Autodesk Inventor part; units mm, degrees
ref_plane "YZ Plane" through (0, 0, 0) normal (1, 0, 0) x (0, 1, 0)
ref_plane "XZ Plane" through (0, 0, 0) normal (0, 1, 0) x (-1, 0, 0)
ref_plane "XY Plane" through (0, 0, 0) normal (0, 0, 1) x (1, 0, 0)
sketch "スケッチ1" plane through (0, 0, 0) normal (0, 0, 1) x (1, 0, 0)
  arc A0 (-5.1, 0) -> (5.1, 0) centre (0, 0) ccw
  line L0 (-15, 8) -> (15, 8)
  line L1 (15, 8) -> (15, 0)
  line L2 (15, 0) -> (5.1, 0)
  line L3 (-15, 0) -> (-15, 8)
  arc A1 (5.1, 0) -> (-5.1, 0) centre (0, 0) ccw
  line L4 (5.1, 0) -> (-5.1, 0)
  line L5 (-5.1, 0) -> (-15, 0)
  dimension "d0" = 10.2
  dimension "d1" = 30
  dimension "d2" = 15
  dimension "d3" = 8
  dimension "d4" = 0
extrude "押し出し1" add sketch "スケッチ1" along normal blind 30 contours L5 L3 L0 L1 L2 A1
sketch "スケッチ2" plane through (-15, 0, 0) normal (0, -1, 0) x (1, 0, 0)
  line L0 (9.9, 30) -> (0, 30)
  line L1 (0, 0) -> (9.9, 0)
  line L2 (0, 30) -> (4.95, 30)
  line L3 (4.95, 30) -> (4.95, 0)
  line L4 (4.95, 0) -> (0, 0)
  line L5 (0, 0) -> (0, 30)
  line L6 (30, 30) -> (25.05, 30)
  line L7 (25.05, 30) -> (25.05, 0)
  line L8 (25.05, 0) -> (30, 0)
  line L9 (30, 0) -> (30, 30)
  line L10 (4.95, 30) -> (9.9, 30)
  line L11 (9.9, 30) -> (9.9, 0)
  line L12 (9.9, 0) -> (4.95, 0)
  line L13 (4.95, 0) -> (4.95, 30)
  line L14 (25.05, 30) -> (20.1, 30)
  line L15 (20.1, 30) -> (20.1, 0)
  line L16 (20.1, 0) -> (25.05, 0)
  line L17 (25.05, 0) -> (25.05, 30)
  point P0 (15, 0)
  dimension "d7" = 30
  dimension "d8" = 4.95
  dimension "d34" = 4.95
extrude "押し出し2" add sketch "スケッチ2" along normal blind 2 contours L11 L1 L3 L0 | L7 L16 L15 L14
fillet "フィレット2" radius 1 4 edges at (-10.05, 0, 15) (-10.05, -2, 15) (10.05, 0, 15) (10.05, -2, 15)
sketch "スケッチ3" plane through (-15, 8, 0) normal (0, 1, 0) x (1, 0, 0)
  line L0 (0, -30) -> (30, -30)
  line L1 (30, 0) -> (30, -30)
  line L2 (30, 0) -> (0, 0)
  line L3 (0, 0) -> (0, -30)
  point P0 (15, 0)
  point P1 (5, -5)
  point P2 (5, -25)
  point P3 (25, -25)
  point P4 (25, -5)
  dimension "d11" = 5
  dimension "d12" = 5
  dimension "d13" = 5
  dimension "d14" = 5
  dimension "d15" = 5
  dimension "d16" = 5
  dimension "d17" = 5
  dimension "d18" = 5
hole "Hole3" at (-10, 8, 5) at (-10, 8, 25) at (10, 8, 25) at (10, 8, 5) direction (0, -1, 0) diameter 3 end through all
sketch "スケッチ4" plane through (0, 0, 30) normal (0, 0, 1) x (1, 0, 0)
  arc A0 (9.05, -2) -> (10.05, -1) centre (9.05, -1) ccw
  arc A1 (11.05, 0) -> (10.05, -1) centre (11.05, -1) ccw
  line L0 (15, 0) -> (11.05, 0)
  line L1 (15, 8) -> (15, 0)
  line L2 (-15, 8) -> (15, 8)
  line L3 (-15, 0) -> (-15, 8)
  line L4 (-11.05, 0) -> (-15, 0)
  arc A2 (-10.05, -1) -> (-11.05, 0) centre (-11.05, -1) ccw
  arc A3 (-10.05, -1) -> (-9.05, -2) centre (-9.05, -1) ccw
  line L5 (-9.05, -2) -> (-5.1, -2)
  line L6 (-5.1, 0) -> (-5.1, -2)
  arc A4 (5.1, 0) -> (-5.1, 0) centre (0, 0) ccw
  line L7 (5.1, 0) -> (5.1, -2)
  line L8 (5.1, -2) -> (9.05, -2)
  line L9 (-15, 0.1) -> (-10.95, 0.1)
  line L10 (-9.95, -0.9) -> (-9.95, -0.9)
  line L11 (-8.95, -1.9) -> (-5.1, -1.9)
  arc A5 (-9.95, -0.9) -> (-10.95, 0.1) centre (-10.95, -0.9) ccw
  arc A6 (-9.95, -0.9) -> (-8.95, -1.9) centre (-8.95, -0.9) ccw
  line L12 (0, 0) -> (0, 8)
  line L13 (15, 0.1) -> (10.95, 0.1)
  line L14 (8.95, -1.9) -> (5.1, -1.9)
  arc A7 (10.95, 0.1) -> (9.95, -0.9) centre (10.95, -0.9) ccw
  arc A8 (8.95, -1.9) -> (9.95, -0.9) centre (8.95, -0.9) ccw
  point P0 (-9.95, 0.1)
  dimension "d43" = 5.05
  dimension "d44" = 2.1
  dimension "d45" = 0.1
  dimension "d46" = 1
equation "\"d34\" = d8"
properties part number "poleHolderB" material "Aluminum-6061"
The listing builds one solid part. Answer for the finished solid, in the listing's coordinates (mm). A direction names the side the tool comes from. Round coordinates to 2 decimals unless told otherwise and drop trailing zeros. Order: outer loops, then holes, each group sorted by start corner. A loop starts at its lowest first (then second) coordinate and runs counter-clockwise, first axis right, second up. Notation, with made-up numbers: (-27.5, 38.5) - (6.5, 38.5) arc R27 cw to (6.5, 57.5) - close; hole circle Ø9 at (71, 16.5). An arc over 180 degrees is marked (long way). Put each result on its own line as item: value. Start each with the question number.
(1) Find section A-A (z = 5). Give the vertices of the cut face in (x, y).
(2) Straight lines are drawn through the part: probe 1 along X at (y, z) = (5.5, 5); probe 2 along Z at (x, y) = (-10, 5.5); probe 3 along X at (y, z) = (-1, 15.5). For each, find the intervals that lie inside material, in ascending order. Write a range as from..to.
(3) Find section B-B (y = 1). Give the vertices of the cut face in (x, z), plus the area to 3 significant figures.
(4) Given P1, Ø2.5, axis at x = 10, z = 25, coming from the -Y side; P2, Ø1.6, axis at y = -1, z = 9, coming from the -X side; P3, Ø4, axis at x = 1, z = 9.5, coming from the -Y side; P4, Ø1.2, axis at x = -14, z = 20.5, coming from the -Y side, each flat-ended and moving along its own axis, determine where each tip first touches the part or whether it passes through.
(5) Determine the mould class of faces 1 (the flat face through (-7, -2, 15)), 2 (the cylindrical face through (-0.1, 5.1, 14.8)), 3 (the cylindrical face through (9.765, -1.699, 14.876)) for opening direction X: released by +X, released by -X, zero draft, split by the parting line, or undercut.
(6) Find section C-C (y = 5.5). Give the vertices of the cut face in (x, z), plus the area to 3 significant figures.
(7) For faces 4 (the cylindrical face through (8.513, 2.93, 4.805)), 5 (the flat face through (-13, 0, 15)), determine the directions among +Z, -Z, +X, -X, +Y, -Y from which every point of the face is accessible in a straight line to the end or side of a thin tool.
Reply:
1. outline: (-15, 0) - (-11.5, 0) - (-11.5, 8) - (-15, 8) - close; (-8.5, -2) - (-5.1, -2) - (-5.1, 0) arc R5.1 cw to (5.1, 0) - (5.1, -2) - (8.5, -2) - (8.5, 8) - (-8.5, 8) - close; (11.5, 0) - (15, 0) - (15, 8) - (11.5, 8) - close
2. probe 1: -15..-11.5, -8.5..8.5, 11.5..15
2. probe 2: 0..3.5, 6.5..23.5, 26.5..30
2. probe 3: -10.05..-5.1, 5.1..10.05
3. outline: (-15, 0) - (-5, 0) - (-5, 30) - (-15, 30) - close; (5, 0) - (15, 0) - (15, 30) - (5, 30) - close; hole circle Ø3 at (-10, 5); hole circle Ø3 at (-10, 25); hole circle Ø3 at (10, 5); hole circle Ø3 at (10, 25)
3. area: 572 mm^2
4. P1: through
4. P2: x = -10.45
4. P3: y = 4.12
4. P4: y = 0
5. face 1: zero draft
5. face 2: undercut
5. face 3: released by +X
6. outline: (-15, 0) - (15, 0) - (15, 30) - (-15, 30) - close; hole circle Ø3 at (-10, 5); hole circle Ø3 at (-10, 25); hole circle Ø3 at (10, 5); hole circle Ø3 at (10, 25)
6. area: 872 mm^2
7. face 4: +Y, -Y
7. face 5: +Z, -Z, -X, -Y
